Part model, mm, in its own coordinate system. Face numbers are marked on the shaded views. A direction names the side the tool comes from. Round coordinates to 2 decimals unless told otherwise and drop trailing zeros. Write each loop counter-clockwise with the first axis right and the second up, starting at its lowest first coordinate (ties: lowest second). Pieces come first, ordered by that corner, then holes.
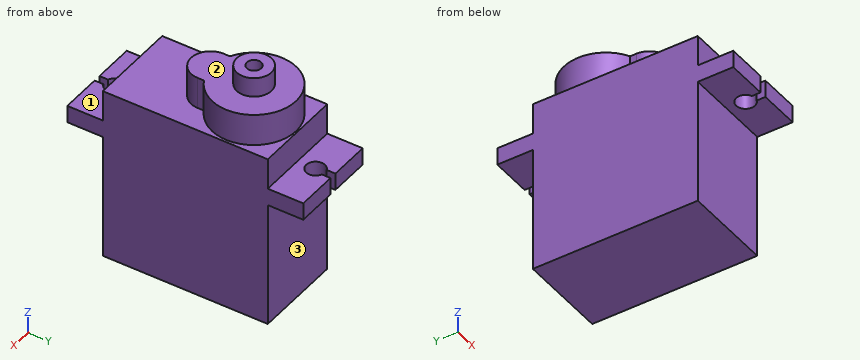
Autodesk Inventor part; units mm, degrees
ref_plane "YZ Plane" through (0, 0, 0) normal (1, 0, 0) x (0, 1, 0)
ref_plane "XZ Plane" through (0, 0, 0) normal (0, 1, 0) x (-1, 0, 0)
ref_plane "XY Plane" through (0, 0, 0) normal (0, 0, 1) x (1, 0, 0)
sketch "Sketch1" plane through (0, 0, 0) normal (0, 0, 1) x (1, 0, 0)
  line L0 (6.15, -11.4) -> (-6.15, -11.4)
  line L1 (-6.15, -11.4) -> (-6.15, 11.4)
  line L2 (-6.15, 11.4) -> (6.15, 11.4)
  line L3 (6.15, 11.4) -> (6.15, -11.4)
  line L4 (6.15, -11.4) -> (-6.15, 11.4) construction
  line L5 (-6.15, -11.4) -> (6.15, 11.4) construction
  line L6 (-6.15, 11.4) -> (-6.15, 16.3)
  line L7 (6.15, 16.3) -> (6.15, 11.4)
  line L8 (-6.15, -11.4) -> (-6.15, -16.3)
  line L9 (6.15, -16.3) -> (6.15, -11.4)
  arc A0 (-0.5, 15.1) -> (0.5, 15.1) centre (0, 13.9) ccw
  line L10 (0, 13.9) -> (0, 11.4) construction
  line L11 (-0.5, 16.3) -> (-0.5, 15.1)
  line L12 (0.5, 15.1) -> (0.5, 16.3)
  line L13 (-0.5, 15.1) -> (0.5, 15.1) construction
  line L14 (0, 13.9) -> (0, 15.1) construction
  line L15 (-6.15, 16.3) -> (-0.5, 16.3)
  line L16 (0.5, 16.3) -> (6.15, 16.3)
  arc A1 (0.5, -15.1) -> (-0.5, -15.1) centre (0, -13.9) ccw
  line L17 (-0.5, -15.1) -> (-0.5, -16.3)
  line L18 (0.5, -15.1) -> (0.5, -16.3)
  line L19 (-0.5, -15.1) -> (0.5, -15.1) construction
  line L20 (0, -15.1) -> (0, -13.9) construction
  line L21 (0, -13.9) -> (0, -11.4) construction
  line L22 (-6.15, -16.3) -> (-0.5, -16.3)
  line L23 (0.5, -16.3) -> (6.15, -16.3)
  line L24 (0, 11.4) -> (0, 5.4) construction
  circle A2 centre (0, 5.4) radius 1
  circle A3 centre (0, 5.4) radius 2.4
  arc A4 (-2.7, -0.6) -> (2.7, -0.6) centre (0, -0.6) ccw
  line L25 (0, 5.4) -> (0, -0.6) construction
  line L26 (-2.7, -0.6) -> (-2.7, 0.2668)
  line L27 (2.7, -0.6) -> (2.7, 0.2668)
  arc A5 (2.7, 0.2668) -> (-2.7, 0.2668) centre (0, 5.4) ccw
  point P0 (0, 0)
  dimension "d0" = 22.8
  dimension "d1" = 12.3
  dimension "d4" = 2.6
  dimension "d5" = 2.5
  dimension "d6" = 1
  dimension "d7" = 4.9
  dimension "d8" = 2.5
  dimension "d9" = 1
  dimension "d10" = 2.6
  dimension "d11" = 4.9
  dimension "d14" = 6
  dimension "d15" = 2
  dimension "d16" = 4.8
  dimension "d17" = 5.4
  dimension "d18" = 6
  dimension "d19" = 5.8
extrude "Extrusion1" add sketch "Sketch1" against normal blind 17.4 contours L0 L1 L2 L3 | A2 | A3 | L26 A5 L27 A4
extrude "Extrusion2" add sketch "Sketch1" along normal blind 2.4 contours L9 L23 L18 A1 L17 L22 L8 L0 | L0 L1 L2 L3 | L2 L6 L15 L11 A0 L12 L16 L7 | A2 | A3 | L26 A5 L27 A4
extrude "Extrusion3" add sketch "Sketch1" along normal blind 4.3 from surface at 2.4 contours L0 L1 L2 L3 | A2 | A3 | L26 A5 L27 A4
extrude "Extrusion4" add sketch "Sketch1" along normal blind 4.4 from surface at 6.7 contours A2 | A3 | L26 A5 L27 A4
extrude "Extrusion5" add sketch "Sketch1" along normal blind 2.7 from surface at 11.1 contours A3
equation "\"d8\" = d5"
equation "\"d9\" = d6"
equation "\"d10\" = d4"
equation "\"d11\" = d7"
equation "\"d3\" = d2"
properties part number "SG90 Servo"
Q1. Saw through at D-D, the plane z = -4.5. Write the cut outline in (x, y), and give its area (3 significant figures).
Q2. Saw through at B-B, the plane x = 0. Write the cut outline in (y, z).
Q3. Saw through at A-A, the plane y = 13.9. Write the cut outline in (x, z).
Q4. Wall check: line 1 (Y direction, x = 0, z = 12.6); line 2 (X direction, y = 13.9, z = 0.65); line 3 (Y direction, x = -5.5, z = -11.5). Give the ranges that are in metal, low to high.
Q5. Saw through at C-C, the plane y = -8. Write the cut outline in (x, z).
Q6. Drop flat-ended pins along their axis: P1, Ø3.5, axis at x = 0, y = -13.9, coming from the -Z side; P2, Ø1, axis at x = 5, z = 7, coming from the -Y side; P3, Ø5.5, axis at x = 2, y = -12.5, coming from the +Z side. Give the stop position or say it passes through.
Q7. Tool access for the marked faces 1, 2 and 3: list every direction of +Z, -Z, +X, -X, +Y, -Y with a clear straight run to the whole face (end or side of a thin tool).
Computed:
1. outline: (-6.15, -11.4) - (6.15, -11.4) - (6.15, 11.4) - (-6.15, 11.4) - close
1. area: 280 mm2
2. outline: (-12.6, 0) - (-11.4, 0) - (-11.4, -17.4) - (11.4, -17.4) - (11.4, 0) - (12.6, 0) - (12.6, 2.4) - (11.4, 2.4) - (11.4, 6.7) - (11.2, 6.7) - (11.2, 11.1) - (7.8, 11.1) - (7.8, 13.8) - (6.4, 13.8) - (6.4, 11.1) - (4.4, 11.1) - (4.4, 13.8) - (3, 13.8) - (3, 11.1) - (-3.3, 11.1) - (-3.3, 6.7) - (-11.4, 6.7) - (-11.4, 2.4) - (-12.6, 2.4) - close
3. outline: (-6.15, 0) - (-1.3, 0) - (-1.3, 2.4) - (-6.15, 2.4) - close; (1.3, 0) - (6.15, 0) - (6.15, 2.4) - (1.3, 2.4) - close
4. line 1: y = 3 to 4.4, 6.4 to 7.8
4. line 2: x = -6.15 to -1.3, 1.3 to 6.15
4. line 3: y = -11.4 to 11.4
5. outline: (-6.15, -17.4) - (6.15, -17.4) - (6.15, 6.7) - (-6.15, 6.7) - close
6. P1: stops at z = 0
6. P2: stops at y = -11.4
6. P3: stops at z = 6.7
7. face 1: +Z, +X, -X, -Y
7. face 2: +Z
7. face 3: -Z, +X, -X, +Y
